Design review of the part built by this model. Coordinates are the model's own, in mm. A direction names the side the tool comes from. Coordinates: 2 decimals unless noted, no trailing zeros. Write each loop counter-clockwise with the first axis right and the second up, starting at its lowest first coordinate (ties: lowest second). Pieces come first, ordered by that corner, then holes. Notation, with made-up numbers: (26.5, 20.5) -> (32.5, 20.5) arc R20 cw to (32.5, 27.5) -> close; hole circle Ø8 at (5, 24.25). An arc over 180 degrees is marked (long way). Return JSON: item names as keys, results as strings. Group by question number.
from build123d import *

# Parameters (mm, degrees)
SKETCH1_R           = 4
BOSS_EXTRUDE1_DEPTH = 10
SKETCH3_W           = 25
SKETCH3_H           = 5
CUT_EXTRUDE1_DEPTH  = 46.82575695
HOLE1_D             = 10
HOLE1_CBORE_D       = 18
HOLE1_CBORE_DEPTH   = 2


with BuildPart() as part:
    # Sketch1 → Boss-Extrude1 (new, symmetric)
    with BuildSketch(Plane(origin=(0, 0, 0), x_dir=(1, 0, 0), z_dir=(0, 1, 0))):
        with BuildLine():
            Line((-30, 10), (30, 10))
            ThreePointArc((30, 10), (40, 0), (30, -10))
            Line((30, -10), (-30, -10))
            ThreePointArc((-30, -10), (-40, 0), (-30, 10))
        make_face()
        with Locations(Location((-30, 0, 0), (0, 0, 270))):
            Circle(SKETCH1_R, mode=Mode.SUBTRACT)
        with Locations(Location((30, 0, 0), (0, 0, 270))):
            Circle(SKETCH1_R, mode=Mode.SUBTRACT)
    extrude(amount=BOSS_EXTRUDE1_DEPTH, both=True)

    # Sketch3 → Cut-Extrude1 (cut, through all)
    with BuildSketch(Plane.XY.offset(10)):
        with Locations((27.5, 0)):
            Rectangle(SKETCH3_W, SKETCH3_H)
        with Locations((-27.5, 0)):
            Rectangle(SKETCH3_W, SKETCH3_H)
    extrude(amount=-CUT_EXTRUDE1_DEPTH, mode=Mode.SUBTRACT)

    # Hole1 (through all)
    with Locations(Plane.XY.offset(10)):
        with Locations((0, 0)):
            CounterBoreHole(HOLE1_D / 2, HOLE1_CBORE_D / 2, HOLE1_CBORE_DEPTH)


solid = part.part
Q1. We need section B-B on z = 0. State how many separate pieces and enclosed holes the cut face has, plus the area to 3 significant figures.
Q2. For P1, Ø1.5, axis at y = 0.5, z = 0.5, coming from the -X side; P2, Ø6, axis at y = 3.5, z = 7, coming from the +X side; P3, Ø4, axis at y = 0, z = 1, coming from the +X side, all flat-tipped, find the tip position at first contact; note any pin that passes through.
Q3. Wall thickness on L1, parallel to X at y = -8, z = 0; L2, parallel to Y at x = -31, z = -4.75; L3, parallel to Z at x = -30, y = 5.25: over which ranges is each line inside the solid? List them lowest first.
Q4. We need section D-D on x = -18. Write out the cut boundary in (y, z).
Q5. The part is to be moulded in two halves that separate along Y. For faces 5 (the flat face through (-6, 7, 10)), 6 (the flat face through (1, -10, 0)), 7 (the flat face through (-25, 2.5, 0)), say which applies: +Y half, -Y half, draft (parallel to the pull), parting line (faces both ways), or undercut.
Q6. For faces 1 (the flat face through (25, 2.5, 0)), 2 (the flat face through (-15, 0, 0)), 3 (the cylindrical face through (1.08, -4.88, -1.13)), 4 (the cylindrical face through (-1.172, 8.923, 9.014)), list the 3-axis set-ups (+Z, -Z, +X, -X, +Y, -Y) from which the entire face can be reached by the end or side of a thin tool; tool diameter is ignored.
Q7. We need section A-A on x = 0. Write out the cut boundary in (y, z).
Q8. We need section C-C on y = 0. Write out the cut boundary in (x, z), plus the area to 3 significant figures.
Findings below:
{
 "1": {"separate pieces": "5", "enclosed holes": "1", "area": "1,030 mm^2"},
 "2": {"P1": "stops at x = -15", "P2": "stops at x = 39.17", "P3": "stops at x = 15"},
 "3": {"L1": "x = -40 to -34, -26 to 26, 34 to 40", "L2": "y = -10 to -2.5, 2.5 to 10", "L3": "z = -10 to -4, 4 to 10"},
 "4": {"outline": "(-10, -10) -> (-2.5, -10) -> (-2.5, 10) -> (-10, 10) -> close; (2.5, -10) -> (10, -10) -> (10, 10) -> (2.5, 10) -> close"},
 "5": {"face 5": "draft", "face 6": "-Y half", "face 7": "undercut"},
 "6": {"face 1": "+Z, -Z, +X", "face 2": "+Z, -Z, -X", "face 3": "+Z, -Z", "face 4": "+Z"},
 "7": {"outline": "(-10, -10) -> (-5, -10) -> (-5, 8) -> (-9, 8) -> (-9, 10) -> (-10, 10) -> close; (5, -10) -> (10, -10) -> (10, 10) -> (9, 10) -> (9, 8) -> (5, 8) -> close"},
 "8": {"outline": "(-15, -10) -> (-5, -10) -> (-5, 8) -> (-9, 8) -> (-9, 10) -> (-15, 10) -> close; (5, -10) -> (15, -10) -> (15, 10) -> (9, 10) -> (9, 8) -> (5, 8) -> close", "area": "384 mm^2"}
}
